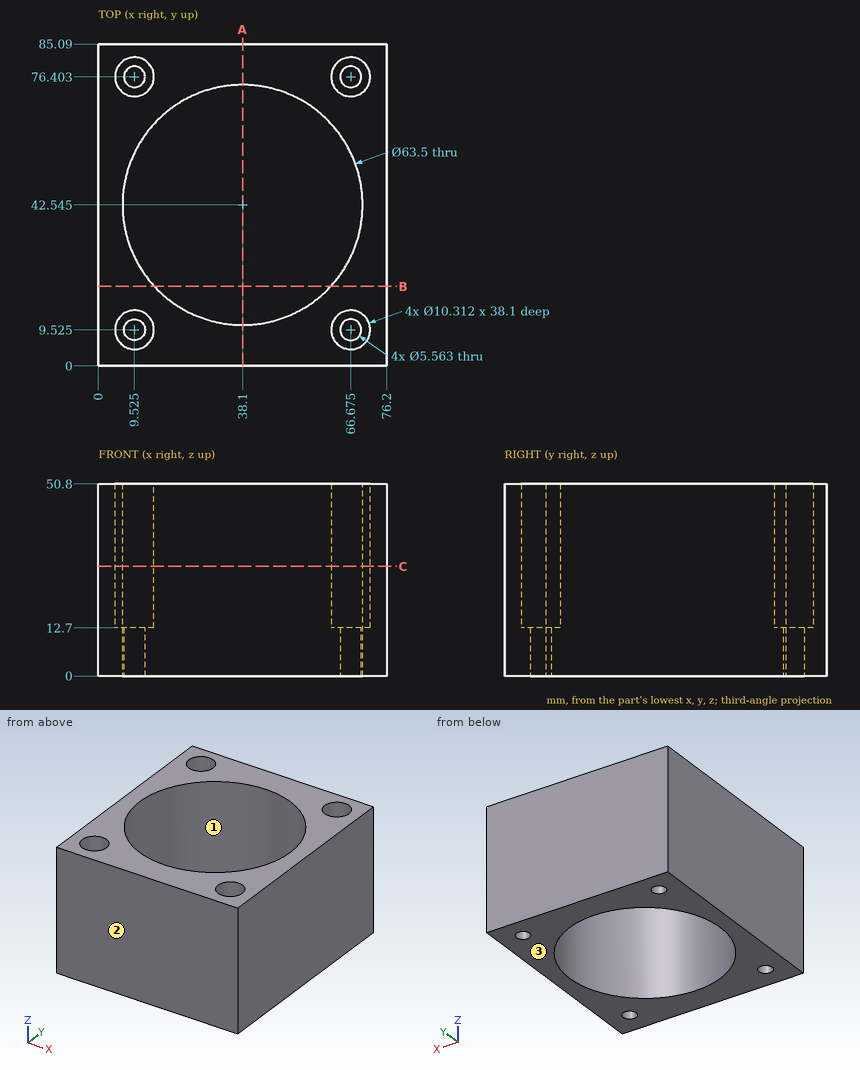
Input: dimensioned drawing with shaded views. Units: mm. Origin: part minimum x, y, z. Give positions to 0.01 mm unless a question says otherwise; leave off trailing zeros. Loops run counter-clockwise (first coordinate to the right, second up) from the corner with the lowest first, then second, coordinate; pieces in that order, holes last. Notation, with made-up numbers: (20, 51) -> (58, 51) arc R18 cw to (58, 75) -> close; hole circle Ø5 at (89, 75). An arc over 180 degrees is marked (long way). Return JSON: item names as keys, results as strings.
Item 1: Line query: line 1 (X direction, y = 64, z = 10) (1 decimal); line 2 (X direction, y = 42, z = 16.5) (1 decimal); line 3 (Y direction, x = 38.1, z = 18.5) (1 decimal). Output: solid intervals per line, ascending.
Filled in:
{"line 1": "0 to 14.7, 61.5 to 76.2", "line 2": "0 to 6.4, 69.8 to 76.2", "line 3": "0 to 10.8, 74.3 to 85.1"}
Item 2: Mould query, pull axis Y, two halves, no side actions, for the marked faces 1, 2 and 3. Classes: released by +Y, released by -Y, zero draft, split by the parting line, or undercut.
Filled in:
{"face 1": "undercut", "face 2": "released by -Y", "face 3": "zero draft"}
Item 3: Pin query (flat end, axial travel): P1, Ø8, axis at x = 65, y = 10, coming from the +Z side; P2, Ø10, axis at x = 14.5, y = 46, coming from the +Z side; P3, Ø3, axis at x = 68.5, y = 76.5, coming from the +Z side. Return the tip coordinate at first contact, or that it passes through.
Filled in:
{"P1": "z = 50.8", "P2": "through", "P3": "z = 12.7"}
Item 4: Section B-B, the plane y = 21. Output: boundary loops of the cut face in (x, z), plus the area to 3 significant figures.
Filled in:
{"outline": "(0, 0) -> (14.78, 0) -> (14.78, 50.8) -> (0, 50.8) -> close; (61.42, 0) -> (76.2, 0) -> (76.2, 50.8) -> (61.42, 50.8) -> close", "area": "1,500 mm^2"}
Item 5: Section A-A, the plane x = 38.1. Output: boundary loops of the cut face in (y, z) (1 decimal).
Filled in:
{"outline": "(0, 0) -> (10.8, 0) -> (10.8, 50.8) -> (0, 50.8) -> close; (74.3, 0) -> (85.1, 0) -> (85.1, 50.8) -> (74.3, 50.8) -> close"}
Item 6: Section C-C, the plane z = 29. Count the separate pieces of the cut face and the enclosed holes in it, plus the area to 3 significant figures.
Filled in:
{"separate pieces": "1", "enclosed holes": "5", "area": "2,980 mm^2"}
